For this review, take the finished solid that the model builds, in its own axes (mm). Face numbers are marked on the shaded views. A direction names the side the tool comes from. Give positions to 0.01 mm unless a question says otherwise; leave off trailing zeros. Order: outer loops, then holes, each group sorted by start corner. A loop starts at its lowest first (then second) coordinate and runs counter-clockwise, first axis right, second up. Notation, with made-up numbers: (36, 59) - (59, 59) arc R14 ccw to (59, 72) - close; hole circle Ø2 at (71, 87). An arc over 180 degrees is marked (long way). Use a Markdown table: item, result. Add a question column.
1) Machinability: for the marked faces 1, 2 and 3, which of the approach directions +Z, -Z, +X, -X, +Y, -Y give a long, thin tool a straight path to every point of the face, cutting with its end or side? Answer none if there is none.
2) Clearance check with flat-ended pins moving along their axes: P1, Ø2, axis at y = 9, z = -1.5, coming from the +X side; P2, Ø0.8, axis at y = 5, z = -0.5, coming from the -X side; P3, Ø1, axis at x = 16.5, y = 8, coming from the +Z side. State where each tip first meets the part, or that it passes through.
3) We need section A-A on x = 20. Write out the cut boundary in (y, z).
4) Wall thickness on L1, parallel to Z at x = 43, y = 2; L2, parallel to X at y = 6.5, z = 2.5; L3, parallel to X at y = 7.75, z = -22.86: over which ranges is each line inside the solid? List them lowest first.
5) We need section C-C on x = -7.5. Write out the cut boundary in (y, z).
6) We need section B-B on y = 6.5. Give the number of separate pieces and of enclosed holes in the cut face, then the cut area to 3 significant figures.
7) We need section D-D on z = -5.5. Write out the cut boundary in (x, y), then the cut area to 3 significant figures.
8) Mouldability with a two-part tool opening along Z and no side actions: class the marked faces 4, 5, 6 and 7 as released by +Z, released by -Z, zero draft, split by the parting line, or undercut.
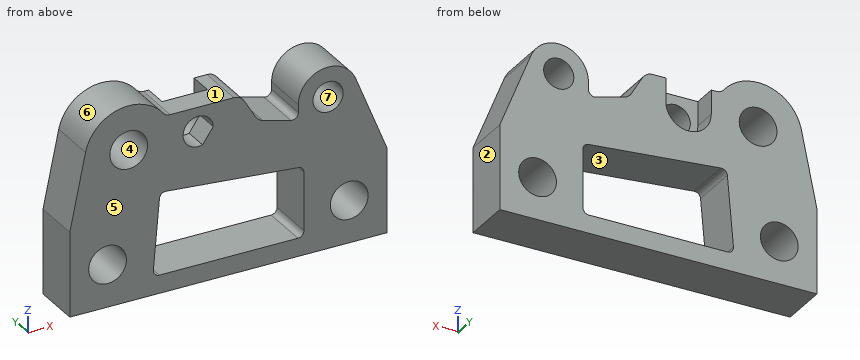
```python
from build123d import *

# Parameters (mm, degrees)
SKETCH3_R           = 3.96875
SKETCH3_R_2         = 3.175
BOSS_EXTRUDE4_DEPTH = 10.16
CUT_EXTRUDE3_DEPTH  = 5.08


with BuildPart() as part:
    # Sketch3 → Boss-Extrude4 (new body)
    with BuildSketch(Plane(origin=(0, 0, 0), x_dir=(1, 0, 0), z_dir=(0, 1, 0))):
        with BuildLine():
            Line((54.2925, 31.75), (-12.3825, 31.75))
            Line((-12.3825, 31.75), (-12.3825, 13.97))
            Line((-12.3825, 13.97), (-9.075895852, -1.891971323))
            ThreePointArc((-9.075895852, -1.891971323), (-2.156945737, -9.016597256), (7.237172055, -5.794375))
            ThreePointArc((7.237172055, -5.794375), (7.899373007, -5.267856205), (8.724262204, -5.08))
            Line((8.724262204, -5.08), (22.098, -5.08))
            ThreePointArc((22.098, -5.08), (23.352279932, -4.748705923), (24.279366546, -3.841245553))
            Line((24.279366546, -3.841245553), (26.647633454, 0.128841561))
            ThreePointArc((26.647633454, 0.128841561), (27.298361404, 0.854600075), (28.174517214, 1.281827513))
            Line((28.174517214, 1.281827513), (34.065158638, 2.852715753))
            ThreePointArc((34.065158638, 2.852715753), (35.166125897, 2.632698945), (35.662400031, 1.6256))
            Line((35.662400031, 1.6256), (35.662400031, 0))
            ThreePointArc((35.662400031, 0), (40.717901726, -6.132813961), (47.702673821, -2.340392141))
            Line((47.702673821, -2.340392141), (54.2925, 13.97))
            Line((54.2925, 13.97), (54.2925, 31.75))
        make_face()
        with Locations(Location((0, 0, 0), (0, 0, 270))):
            Circle(SKETCH3_R, mode=Mode.SUBTRACT)
        with Locations(Location((-4.445, 22.86, 0), (0, 0, 270))):
            Circle(SKETCH3_R, mode=Mode.SUBTRACT)
        with Locations(Location((46.355, 22.86, 0), (0, 0, 270))):
            Circle(SKETCH3_R, mode=Mode.SUBTRACT)
        with Locations(Location((41.91, 0, 0), (0, 0, 270))):
            Circle(SKETCH3_R_2, mode=Mode.SUBTRACT)
        with BuildLine():
            Line((17.774504023, -0.186733089), (15.513562514, 3.04222602))
            ThreePointArc((15.513562514, 3.04222602), (12.004192259, -1.821105185), (17.774504023, -0.186733089))
        make_face(mode=Mode.SUBTRACT)
        with BuildLine():
            Line((36.83, 14.42919116), (36.83, 26.67))
            ThreePointArc((36.83, 26.67), (36.458025612, 27.568025612), (35.56, 27.94))
            Line((35.56, 27.94), (6.442341733, 27.94))
            ThreePointArc((6.442341733, 27.94), (5.505999515, 27.527999564), (5.177174467, 26.559312207))
            Line((5.177174467, 26.559312207), (6.461152869, 11.883371914))
            ThreePointArc((6.461152869, 11.883371914), (6.909979871, 11.021183265), (7.837007929, 10.728892441))
            Line((7.837007929, 10.728892441), (35.670687793, 13.164023894))
            ThreePointArc((35.670687793, 13.164023894), (36.496342218, 13.571191596), (36.83, 14.42919116))
        make_face(mode=Mode.SUBTRACT)
    extrude(amount=BOSS_EXTRUDE4_DEPTH)

    # Sketch5 → Cut-Extrude3 (cut)
    with BuildSketch(Plane(origin=(0, 10.16, 0), x_dir=(1, 0, 0), z_dir=(0, 1, 0))):
        with BuildLine():
            Line((19.3675, 0), (19.3675, -5.08))
            Line((19.3675, -5.08), (9.8425, -5.08))
            Line((9.8425, -5.08), (9.8425, 0))
            ThreePointArc((9.8425, 0), (14.605, 4.7625), (19.3675, 0))
        make_face()
    extrude(amount=-CUT_EXTRUDE3_DEPTH, mode=Mode.SUBTRACT)


solid = part.part
```
Checked values:
| question | item | result |
|---|---|---|
| 1 | face 1 | +Z, +Y, -Y |
| 1 | face 2 | +Z, -Z, +X, +Y, -Y |
| 1 | face 3 | +Y, -Y |
| 2 | P1 | x = 49.66 |
| 2 | P2 | x = -9.66 |
| 2 | P3 | z = -4.12 |
| 3 | outline | (0, -31.75) - (10.16, -31.75) - (10.16, -27.94) - (0, -27.94) - close; (0, -11.79) - (10.16, -11.79) - (10.16, 5.08) - (0, 5.08) - close |
| 4 | L1 | -31.75 to -24.98, -20.74 to -2.98, 2.98 to 6.15 |
| 4 | L2 | -8.93 to -3.08, 3.08 to 9.84, 19.37 to 25.08, 36.18 to 39.95, 43.87 to 47.64 |
| 4 | L3 | -12.38 to -8.41, -0.48 to 5.5, 36.83 to 42.39, 50.32 to 54.29 |
| 5 | outline | (0, -31.75) - (10.16, -31.75) - (10.16, -25.39) - (0, -25.39) - close; (0, -20.33) - (10.16, -20.33) - (10.16, 5.45) - (0, 5.45) - close |
| 6 | separate pieces | 1 |
| 6 | enclosed holes | 5 |
| 6 | area | 1,560 mm² |
| 7 | outline | (-10.62, 0) - (50.87, 0) - (50.87, 10.16) - (-10.62, 10.16) - close |
| 7 | area | 625 mm² |
| 8 | face 4 | undercut |
| 8 | face 5 | zero draft |
| 8 | face 6 | released by +Z |
| 8 | face 7 | undercut |
